from build123d import *

# Parameters (mm, degrees)
F0_W     = 101.6
F0_H     = 203.2
F1_DEPTH = 7.62
F3_DEPTH = 25.4
F4_W     = 21.7
F4_H     = 22.33677
F4_W_2   = 15.7
F4_H_2   = 16.33677
F5_DEPTH = 25.4


with BuildPart() as f1:
    # F0 (on Top) → F1 (new body)
    with BuildSketch(Plane.XY):
        Rectangle(F0_W, F0_H)
    extrude(amount=F1_DEPTH)

    # F2 (on Top) → F3 (cut)
    with BuildSketch(Plane.XY):
        with BuildLine():
            Line((-15.035691, -77.822713), (-14.988321, -81.421245))
            ThreePointArc((-14.988321, -81.421245), (-13.081192, -83.592345), (-11.008666, -81.578528))
            Line((-11.008666, -81.578528), (-11.048887, -77.843856))
            ThreePointArc((-11.048887, -77.843856), (-13.031485, -75.796128), (-15.035691, -77.822713))
        make_face()
        with BuildLine():
            ThreePointArc((-15.035691, -95.377287), (-13.031485, -97.403872), (-11.048887, -95.356144))
            Line((-11.048887, -95.356144), (-11.008666, -91.621472))
            ThreePointArc((-11.008666, -91.621472), (-13.081192, -89.607655), (-14.988321, -91.778755))
            Line((-14.988321, -91.778755), (-15.035691, -95.377287))
        make_face()
        with BuildLine():
            ThreePointArc((15.035691, -77.822713), (13.031485, -75.796128), (11.048887, -77.843856))
            Line((11.048887, -77.843856), (11.008666, -81.578528))
            ThreePointArc((11.008666, -81.578528), (13.081192, -83.592345), (14.988321, -81.421245))
            Line((14.988321, -81.421245), (15.035691, -77.822713))
        make_face()
        with BuildLine():
            Line((11.008666, -91.621472), (11.048887, -95.356144))
            ThreePointArc((11.048887, -95.356144), (13.031485, -97.403872), (15.035691, -95.377287))
            Line((15.035691, -95.377287), (14.988321, -91.778755))
            ThreePointArc((14.988321, -91.778755), (13.081192, -89.607655), (11.008666, -91.621472))
        make_face()
        with BuildLine():
            ThreePointArc((15.035691, 95.377287), (13.031485, 97.403872), (11.048887, 95.356144))
            Line((11.048887, 95.356144), (11.008666, 91.621472))
            ThreePointArc((11.008666, 91.621472), (13.081192, 89.607655), (14.988321, 91.778755))
            Line((14.988321, 91.778755), (15.035691, 95.377287))
        make_face()
        with BuildLine():
            Line((-11.008666, 91.621472), (-11.048887, 95.356144))
            ThreePointArc((-11.048887, 95.356144), (-13.031485, 97.403872), (-15.035691, 95.377287))
            Line((-15.035691, 95.377287), (-14.988321, 91.778755))
            ThreePointArc((-14.988321, 91.778755), (-13.081192, 89.607655), (-11.008666, 91.621472))
        make_face()
        with BuildLine():
            ThreePointArc((-15.035691, 77.822713), (-13.031485, 75.796128), (-11.048887, 77.843856))
            Line((-11.048887, 77.843856), (-11.008666, 81.578528))
            ThreePointArc((-11.008666, 81.578528), (-13.081192, 83.592345), (-14.988321, 81.421245))
            Line((-14.988321, 81.421245), (-15.035691, 77.822713))
        make_face()
        with BuildLine():
            ThreePointArc((11.048887, 77.843856), (13.031485, 75.796128), (15.035691, 77.822713))
            Line((15.035691, 77.822713), (14.988321, 81.421245))
            ThreePointArc((14.988321, 81.421245), (13.081192, 83.592345), (11.008666, 81.578528))
            Line((11.008666, 81.578528), (11.048887, 77.843856))
        make_face()
    extrude(amount=F3_DEPTH, mode=Mode.SUBTRACT)

    # F4 (on face) → F5 (join)
    with BuildSketch(Plane.XY.offset(7.62)):
        with Locations((38.1, 88.9)):
            Rectangle(F4_W, F4_H)
        with Locations((38.1, 88.9)):
            Rectangle(F4_W_2, F4_H_2, mode=Mode.SUBTRACT)
        with Locations((38.1, -88.9)):
            Rectangle(F4_W, F4_H)
        with Locations((38.1, -88.9)):
            Rectangle(F4_W_2, F4_H_2, mode=Mode.SUBTRACT)
        with Locations((-38.1, 88.9)):
            Rectangle(F4_W, F4_H)
        with Locations((-38.1, 88.9)):
            Rectangle(F4_W_2, F4_H_2, mode=Mode.SUBTRACT)
        with Locations((-38.1, -88.9)):
            Rectangle(F4_W, F4_H)
        with Locations((-38.1, -88.9)):
            Rectangle(F4_W_2, F4_H_2, mode=Mode.SUBTRACT)
    extrude(amount=F5_DEPTH)


solid = f1.part
Check sheet for the modelled part. Datum: model origin and axes. Units: mm. A direction names the side the tool comes from. Round coordinates to 2 decimals unless told otherwise and drop trailing zeros. Loops run counter-clockwise (first coordinate to the right, second up) from the corner with the lowest first, then second, coordinate; pieces in that order, holes last. Notation, with made-up numbers: M -31,78 L 23,78 A25 ccw 23,115 Z; hole C 82,34.25 d2. An arc over 180 degrees is marked long. One line per question, with ' | ' between items. Start each with the question number.
Item 1: Scan lines: probe 1 along X at (y, z) = (-82, 15.5); probe 2 along Y at (x, z) = (-43, 20); probe 3 along Z at (x, y) = (-4.5, 89.5). Record each from-to range of solid material in increasing order.
Item 2: Section check B-B (y = 10.5). Record the boundary of the cut face in (x, z), and give its area (3 significant figures).
Item 3: Release check for a two-part mould opening along X. For faces 1 (the face through (48, -89, 33.02)), 2 (the face through (48.95, 89, 20)), 3 (the face through (-30.25, -89, 20)) record: released by +X, released by -X, zero draft, split by the parting line, or undercut.
Item 4: Gauge pin test, flat ends, axial feed: pin 1 Ø4.5 at (x, z) = (-40, 20.5) entering from -Y; pin 2 Ø18 at (y, z) = (-90, 20) entering from -X; pin 3 Ø18 at (y, z) = (93.5, 20.5) entering from +X. Record the tip position at first contact, or that the pin passes through.
Item 5: Section check A-A (z = 14.5). State how many separate pieces and enclosed holes the cut face has, and give its area (3 significant figures).
Item 6: Set-up check for faces 4 (the face through (50.8, -1, 4)), 5 (the face through (27.25, 89, 20)), 6 (the face through (30.25, 89, 20)), 7 (the face through (13.13, 83.59, 3.76)), 8 (the face through (38, -77.732, 20)): record each of +Z, -Z, +X, -X, +Y, -Y from which the full face is reachable in a straight line by a thin tool's end or side.
Worked out:
1) probe 1: -48.95 to -45.95, -30.25 to -27.25, 27.25 to 30.25, 45.95 to 48.95 | probe 2: -100.07 to -97.07, -80.73 to -77.73, 77.73 to 80.73, 97.07 to 100.07 | probe 3: 0 to 7.62
2) outline: M -50.8,0 L 50.8,0 L 50.8,7.62 L -50.8,7.62 Z | area: 774 mm^2
3) face 1: zero draft | face 2: released by +X | face 3: undercut
4) pin 1: y = -100.07 | pin 2: x = -48.95 | pin 3: x = 48.95
5) separate pieces: 4 | enclosed holes: 4 | area: 913 mm^2
6) face 4: +Z, -Z, +X, +Y, -Y | face 5: +Z, +Y, -Y | face 6: +Z | face 7: +Z, -Z | face 8: +Z, +X, -X
